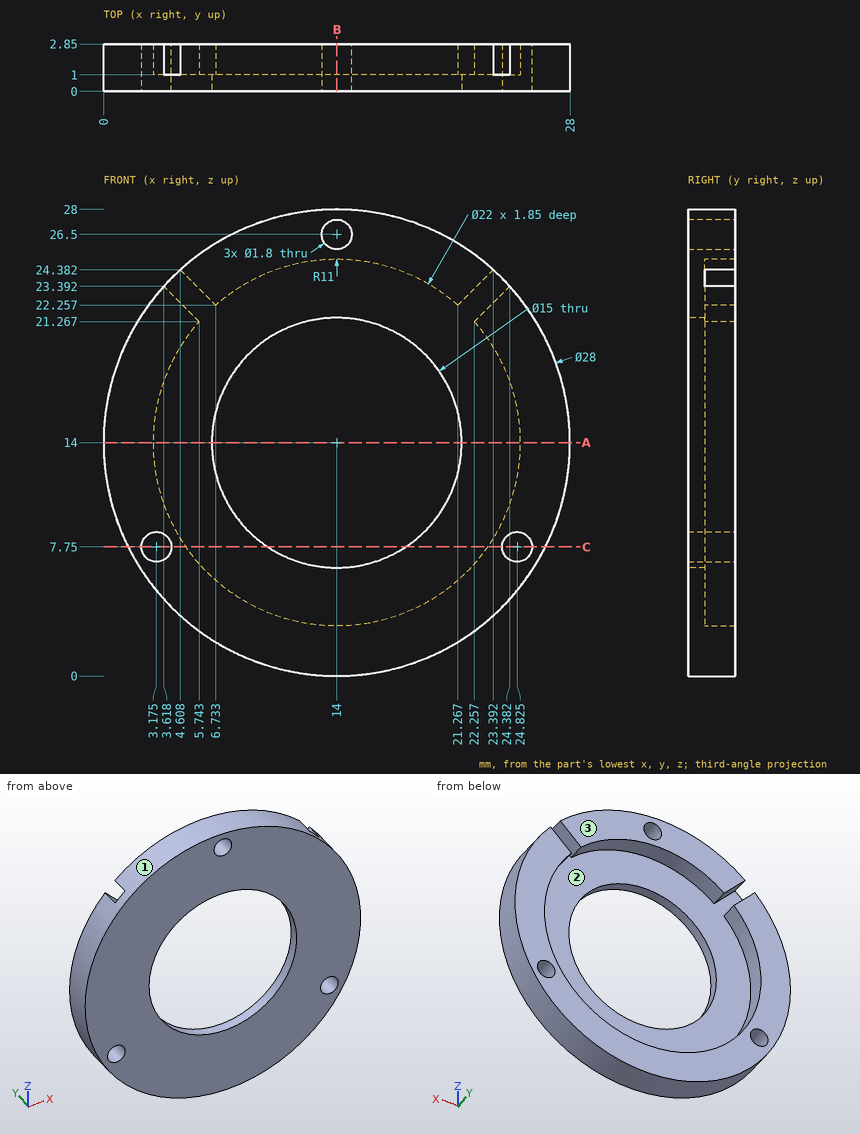
Verification items for this drawing (mm, ordinates from the low corner). Give positions to 0.01 mm unless a question says otherwise; leave off trailing zeros. Loops run counter-clockwise (first coordinate to the right, second up) from the corner with the lowest first, then second, coordinate; pieces in that order, holes last. Notation, with made-up numbers: M 88,-22.5 L 131,-22.5 A21 ccw 131,10.5 Z; hole C -20,-23.75 d4. An arc over 180 degrees is marked long. Return JSON: item names as keys, results as strings. Group by question number.
1. Cross-section at B-B on x = 14. Record the boundary of the cut face in (y, z).
2. Cross-section at C-C on z = 7.75. State how many separate pieces and enclosed holes the cut face has.
3. Cross-section at A-A on z = 14. Record the boundary of the cut face in (x, y).
4. Thickness scan on L1, parallel to Z at x = 14, y = 1.85; L2, parallel to Z at x = 14, y = 0.4; L3, parallel to X at y = 0.4, z = 18 (1 decimal). Record the ranges inside material, lowest first.
5. Go/stop test with a flat-tipped pin: pin 1 (1.5 mm diameter, centred on x = 12.5, y = 1, fed in from +Z). Record where the tip stops, or that it passes through.
6. Mould release check, pull along Z, two halves, no side actions. Record for the marked faces 1, 2 and 3: released by +Z, released by -Z, zero draft, split by the parting line, or undercut.
Return value:
{
 "1": {"outline": "M 0,0 L 2.85,0 L 2.85,3 L 1,3 L 1,6.5 L 0,6.5 Z; M 0,21.5 L 1,21.5 L 1,25 L 2.85,25 L 2.85,25.6 L 0,25.6 Z; M 0,27.4 L 2.85,27.4 L 2.85,28 L 0,28 Z"},
 "2": {"separate pieces": "4", "enclosed holes": "0"},
 "3": {"outline": "M 0,0 L 6.5,0 L 6.5,1 L 3,1 L 3,2.85 L 0,2.85 Z; M 21.5,0 L 28,0 L 28,2.85 L 25,2.85 L 25,1 L 21.5,1 Z"},
 "4": {"L1": "0 to 3, 25 to 25.6, 27.4 to 28", "L2": "0 to 6.5, 21.5 to 25.6, 27.4 to 28", "L3": "0.6 to 7.7, 20.3 to 27.4"},
 "5": {"pin 1": "z = 27.98"},
 "6": {"face 1": "split by the parting line", "face 2": "undercut", "face 3": "zero draft"}
}
